The model under review builds one solid part; all positions refer to its coordinate system, in mm. Face numbers are marked on the shaded views. A direction names the side the tool comes from. Coordinates: 2 decimals unless noted, no trailing zeros. Write each loop counter-clockwise with the first axis right and the second up, starting at its lowest first coordinate (ties: lowest second). Pieces come first, ordered by that corner, then holes. Notation, with made-up numbers: M 75,-22.75 L 109,-22.75 A21 ccw 109,-10.75 Z; hole C -40,1 d7. An arc over 180 degrees is marked long. Answer as a JSON object with one key per item and string values.
```python
from build123d import *

# Parameters (mm, degrees)
F0_W     = 47.9057580233
F0_H     = 73.8517567515
F1_DEPTH = 76.2
F3_DEPTH = 73.7290531397
F4_W     = 7.8228898346
F4_H     = 14.375641942
F4_W_2   = 8.3178766072
F4_H_2   = 14.0072628856
F4_W_3   = 6.03377074
F4_H_3   = 28.6656171083
F5_DEPTH = 6.5299868584
F6_W     = 10.6063969433
F6_H     = 13.3831351995
F6_H_2   = 12.8184799105
F6_W_2   = 10.7133537531
F7_DEPTH = 25.4


with BuildPart() as f1:
    # F0 (on Top) → F1 (new body)
    with BuildSketch(Plane.XY):
        with Locations((23.9528790116, 14.6708004177)):
            Rectangle(F0_W, F0_H)
    extrude(amount=F1_DEPTH)

    # F2 (on face) → F3 (join)
    with BuildSketch(Plane.XZ.offset(22.2550779581)):
        Polygon((37.7622656524, 159.051656723), (-20.4486101866, 71.3405758142), (0, 71.3405758142), (0, 76.2), (47.9057580233, 76.2), (47.9057580233, 71.3405758142), (77.7672529221, 71.3405758142), align=None)
    extrude(amount=-F3_DEPTH)

    # F4 (on face) → F5 (cut)
    with BuildSketch(Plane.XZ.offset(22.2550779581)):
        with Locations((11.8029844016, 53.7293627858)):
            Rectangle(F4_W, F4_H)
        with Locations((34.3761388212, 54.1785098612)):
            Rectangle(F4_W_2, F4_H_2)
        with Locations((20.9359936416, 14.3328085542)):
            Rectangle(F4_W_3, F4_H_3)
    extrude(amount=-F5_DEPTH, mode=Mode.SUBTRACT)

    # F6 (on face) → F7 (cut)
    with BuildSketch(Plane.YZ.offset(47.9057580233)):
        with Locations((-5.3031984717, 53.1773492694)):
            Rectangle(F6_W, F6_H)
        with Locations((-5.3031984717, 24.7165327892)):
            Rectangle(F6_W, F6_H_2)
        with Locations((27.5034122169, 24.7165327892)):
            Rectangle(F6_W_2, F6_H_2)
        with Locations((27.5034122169, 53.1773492694)):
            Rectangle(F6_W_2, F6_H)
    extrude(amount=-F7_DEPTH, mode=Mode.SUBTRACT)


solid = f1.part
```
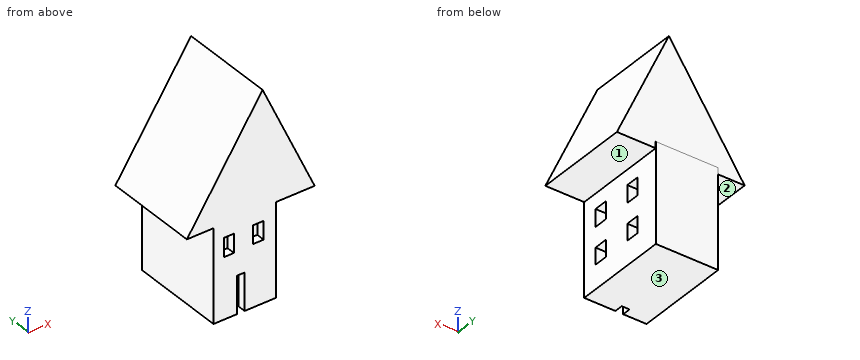
(1) For the marked faces 1, 2 and 3, list the 3-axis set-ups (+Z, -Z, +X, -X, +Y, -Y) from which the entire face can be reached by the end or side of a thin tool; tool diameter is ignored.
Results list:
{"face 1": "-Z, +X, +Y, -Y", "face 2": "-Z, -X, +Y, -Y", "face 3": "-Z, +X, -X, +Y, -Y"}
(2) Add section C-C on y = -2. Give the boundary of the cut face in (x, z), and give its area (3 significant figures).
Results list:
{"outline": "M -20.45,71.34 L 0,71.34 L 0,0 L 47.91,0 L 47.91,18.31 L 22.51,18.31 L 22.51,31.13 L 47.91,31.13 L 47.91,46.49 L 22.51,46.49 L 22.51,59.87 L 47.91,59.87 L 47.91,71.34 L 77.77,71.34 L 37.76,159.05 Z", "area": "7,060 mm²"}
(3) For pin 1 Ø3.5 at (x, y) = (11, -20.5) entering from +Z; pin 2 Ø6.5 at (x, z) = (35.5, 55) entering from -Y; pin 3 Ø22.5 at (x, y) = (-13, 12.5) entering from -Z; pin 4 Ø5 at (y, z) = (2.5, 43.5) entering from -X, all flat-tipped, find the tip position at first contact; note any pin that passes through.
Results list:
{"pin 1": "z = 121.36", "pin 2": "y = -22.26", "pin 3": "z = 71.34", "pin 4": "x = 0"}
(4) Add section D-D on x = 53.5. Give the boundary of the cut face in (y, z), and give its area (3 significant figures).
Results list:
{"outline": "M -22.26,71.34 L 51.47,71.34 L 51.47,124.55 L -22.26,124.55 Z", "area": "3,920 mm²"}
(5) Add section A-A on y = 36. Give the boundary of the cut face in (x, z).
Results list:
{"outline": "M -20.45,71.34 L 0,71.34 L 0,0 L 47.91,0 L 47.91,71.34 L 77.77,71.34 L 37.76,159.05 Z"}
(6) Add section B-B on z = 53. Give the boundary of the cut face in (x, y).
Results list:
{"outline": "M 0,-22.26 L 7.89,-22.26 L 7.89,-15.73 L 15.71,-15.73 L 15.71,-22.26 L 30.22,-22.26 L 30.22,-15.73 L 38.54,-15.73 L 38.54,-22.26 L 47.91,-22.26 L 47.91,-10.61 L 22.51,-10.61 L 22.51,0 L 47.91,0 L 47.91,22.15 L 22.51,22.15 L 22.51,32.86 L 47.91,32.86 L 47.91,51.6 L 0,51.6 Z"}
(7) Wall thickness on line 1 along Y through (x, z) = (29, 54); line 2 along Y through (x, z) = (40, 112); line 3 along Z through (x, y) = (36, -8.5): over which ranges is each line inside the solid? List them lowest first. Write a range as from..to.
Results list:
{"line 1": "-22.26..-10.61, 0..22.15, 32.86..51.6", "line 2": "-22.26..51.47", "line 3": "0..18.31, 31.13..46.49, 59.87..156.4"}
